```python
from build123d import *

# Parameters (mm, degrees)
SKETCH1_W                   = 40
SKETCH1_H                   = 40
BOSS_EXTRUDE1_DEPTH         = 2
BOSS_EXTRUDE2_DEPTH         = 73
BOSS_EXTRUDE2_DEPTH_BACK    = 2
SKETCH2_W                   = 40
SKETCH2_H                   = 1
FILLET1_R                   = 1
SKETCH4_R                   = 2.25
SKETCH4_W                   = 0.5
SKETCH4_H                   = 6.8
CUT_EXTRUDE1_DEPTH          = 49
M3_TAPPED_HOLE1_D           = 2.5
M3_TAPPED_HOLE1_CSINK_D     = 3.05
M3_TAPPED_HOLE1_CSINK_ANGLE = 90


with BuildPart() as part:
    # Sketch1 → Boss-Extrude1 (new body)
    with BuildSketch(Plane(origin=(0, 0, 0), x_dir=(1, 0, 0), z_dir=(0, 1, 0))):
        with Locations((20, 20)):
            Rectangle(SKETCH1_W, SKETCH1_H)
    extrude(amount=BOSS_EXTRUDE1_DEPTH)

    # Sketch2 → Boss-Extrude2 (add, two sides: drawn at the far end of the back side and taken through both)
    with BuildSketch(Plane(origin=(0, 2, 0), x_dir=(1, 0, 0), z_dir=(0, 1, 0)).offset(-BOSS_EXTRUDE2_DEPTH_BACK)):
        with Locations((20, 0.5)):
            Rectangle(SKETCH2_W, SKETCH2_H)
        with Locations((20, -0.5)):
            Rectangle(SKETCH2_W, SKETCH2_H)
    extrude(amount=BOSS_EXTRUDE2_DEPTH + BOSS_EXTRUDE2_DEPTH_BACK)

    # Fillet1
    fillet1_edges = [part.edges().sort_by_distance(p)[0] for p in [
        (20, 2, -1),
        (20, 0, 1),
    ]]
    fillet(fillet1_edges, radius=FILLET1_R)

    # Sketch4 → Cut-Extrude1 (cut)
    with BuildSketch(Plane.XY.offset(1)):
        with Locations((15, 62.4)):
            Circle(SKETCH4_R)
        with Locations((19.75, 61.6)):
            Rectangle(SKETCH4_W, SKETCH4_H)
        with Locations((20.25, 61.6)):
            Rectangle(SKETCH4_W, SKETCH4_H)
        with Locations((25, 62.4)):
            Circle(SKETCH4_R)
        Polygon((20.5, 58.2), (20, 58.2), (20, 17.8), (20.5, 17.8), (30, 17.8), (30, 58.2), align=None)
        Polygon((20, 17.8), (20, 58.2), (19.5, 58.2), (10, 58.2), (10, 17.8), (19.5, 17.8), align=None)
        with Locations((19.75, 14.4)):
            Rectangle(SKETCH4_W, SKETCH4_H)
        with Locations((15, 13.6)):
            Circle(SKETCH4_R)
        with Locations((20.25, 14.4)):
            Rectangle(SKETCH4_W, SKETCH4_H)
        with Locations((25, 13.6)):
            Circle(SKETCH4_R)
    extrude(amount=-CUT_EXTRUDE1_DEPTH, mode=Mode.SUBTRACT)

    # M3 Tapped Hole1 (through all)
    with Locations(Plane(origin=(0, 2, 0), x_dir=(1, 0, 0), z_dir=(0, 1, 0))):
        with Locations((20, 15)):
            CounterSinkHole(M3_TAPPED_HOLE1_D / 2, M3_TAPPED_HOLE1_CSINK_D / 2, counter_sink_angle=M3_TAPPED_HOLE1_CSINK_ANGLE)


solid = part.part
```
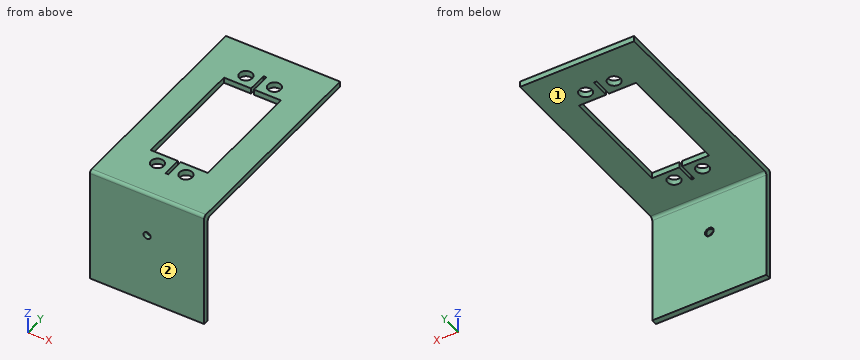
Could you check a few things on this model? Use its own coordinates, in mm. Face numbers are marked on the shaded views. A direction names the side the tool comes from. Round coordinates to 2 decimals unless told otherwise and drop trailing zeros. Loops run counter-clockwise (first coordinate to the right, second up) from the corner with the lowest first, then second, coordinate; pieces in that order, holes last.
Q1. Please list where these lines run through material, in increasing order: L1, parallel to Y at x = 15, z = -0.15; L2, parallel to X at y = 13, z = 0; L3, parallel to Y at x = 8, z = -28.
Q2. For P1, Ø0.6, axis at y = 39, z = 0.5, coming from the -X side; P2, Ø4, axis at x = 25, y = 62.4, coming from the -Z side; P3, Ø11.5, axis at x = 15, z = -28, coming from the +Y side, each with a flat end and sliding along its axis, tell me the tip position at first contact or that it passes through.
Q3. I want a section at B-B (z = -15). Write out the boundary of the cut face in (x, y) (3 decimals), and give its area (3 significant figures).
Q4. I want a section at C-C (x = 25). Write out the boundary of the cut face in (y, z).
Q5. I want a section at D-D (y = 13.6). Write out the boundary of the cut face in (x, z).
Q6. On a 3-axis mill with a long thin cutter (end or side, diameter ignored), from which of +Z, -Z, +X, -X, +Y, -Y can I reach the whole of each face in a straight line? I mean the marked faces 1 and 2. Say none if no direction works.
Q7. I want a section at A-A (y = 50). Write out the boundary of the cut face in (x, z), and give its area (3 significant figures).
Answer below:
1. L1: y = 0 to 11.35, 15.85 to 17.8, 58.2 to 60.15, 64.65 to 75
1. L2: x = 0 to 12.83, 17.17 to 19.5, 20.5 to 22.83, 27.17 to 40
1. L3: y = 0 to 2
2. P1: stops at x = 0
2. P2: passes through
2. P3: stops at y = 2
3. outline: (0, 0) - (18.75, 0) - (18.75, 1.725) - (18.475, 2) - (0, 2) - close; (21.25, 0) - (40, 0) - (40, 2) - (21.525, 2) - (21.25, 1.725) - close
3. area: 74.9 mm2
4. outline: (0, -40) - (2, -40) - (2, -2) arc R1 cw to (3, -1) - (11.35, -1) - (11.35, 1) - (1, 1) arc R1 ccw to (0, 0) - close; (15.85, -1) - (17.8, -1) - (17.8, 1) - (15.85, 1) - close; (58.2, -1) - (60.15, -1) - (60.15, 1) - (58.2, 1) - close; (64.65, -1) - (75, -1) - (75, 1) - (64.65, 1) - close
5. outline: (0, -1) - (12.75, -1) - (12.75, 1) - (0, 1) - close; (17.25, -1) - (19.5, -1) - (19.5, 1) - (17.25, 1) - close; (20.5, -1) - (22.75, -1) - (22.75, 1) - (20.5, 1) - close; (27.25, -1) - (40, -1) - (40, 1) - (27.25, 1) - close
6. face 1: -Z, +X, -X, +Y
6. face 2: +Z, -Z, +X, -X, -Y
7. outline: (0, -1) - (10, -1) - (10, 1) - (0, 1) - close; (30, -1) - (40, -1) - (40, 1) - (30, 1) - close
7. area: 40.0 mm2
